Job drawing, mm, ordinate dimensions from the low corner. One solid piece. A direction names the side the tool comes from. Coordinates: 2 decimals unless noted, no trailing zeros. Order: outer loops, then holes, each group sorted by start corner. A loop starts at its lowest first (then second) coordinate and runs counter-clockwise, first axis right, second up. Notation, with made-up numbers: (26, -26) - (52, -26) arc R18 cw to (52, -2) - close; hole circle Ø6 at (37.25, 11). An arc over 180 degrees is marked (long way). Use one line per item in the form item = value.
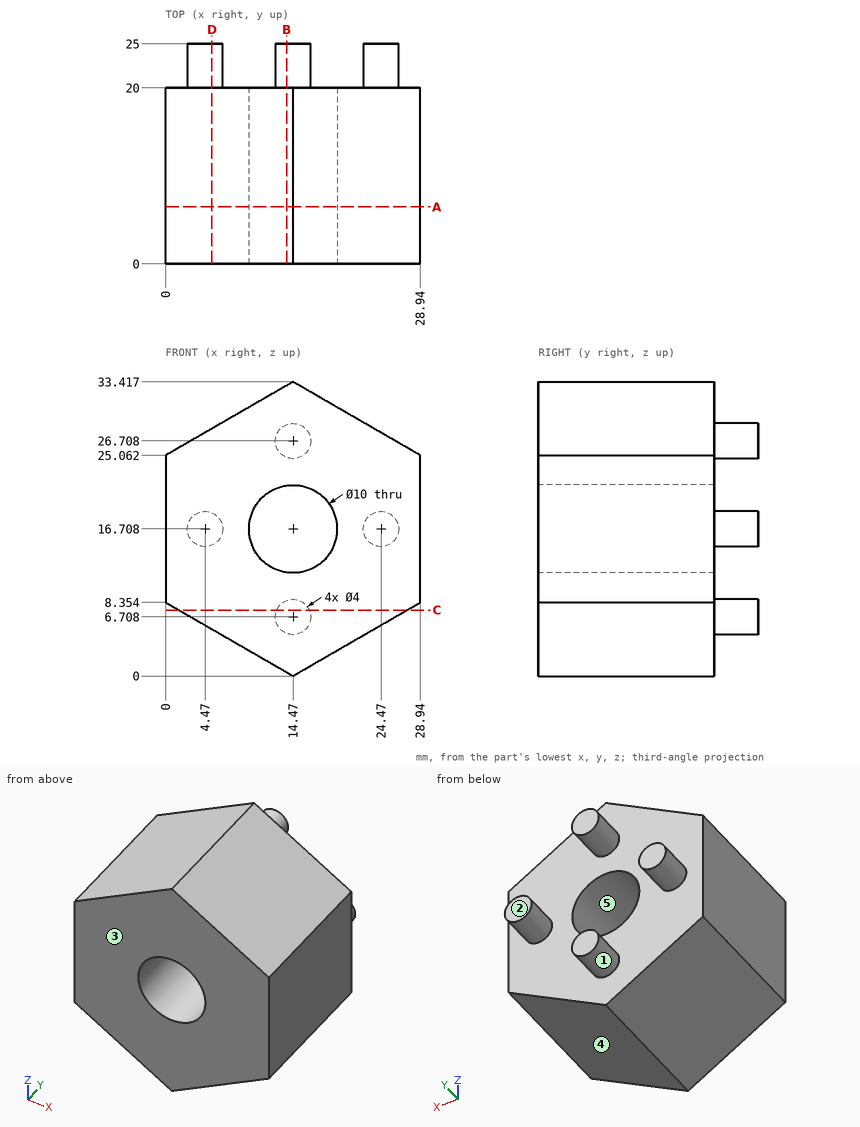
Item 1: Cut at B-B, the plane x = 13.75. Write the cut outline in (y, z) (1 decimal).
Derived:
outline = (0, 0.4) - (20, 0.4) - (20, 4.8) - (25, 4.8) - (25, 8.6) - (20, 8.6) - (20, 11.8) - (0, 11.8) - close; (0, 21.7) - (20, 21.7) - (20, 24.8) - (25, 24.8) - (25, 28.6) - (20, 28.6) - (20, 33) - (0, 33) - close
Item 2: Two-plate mould, pull along Z, no slides. Class the marked faces 3, 4 and 5: +Z half, -Z half, draft (parallel to the pull), parting line (faces both ways), or undercut.
Derived:
face_3 = draft
face_4 = -Z half
face_5 = undercut
Item 3: Drill centre lines: line 1 (Y direction, x = 14.5, z = 31.5); line 2 (Z direction, x = 15.5, y = 10.5) (1 decimal); line 3 (Z direction, x = 24.5, y = 9.5) (1 decimal). Where is each one in solid material? Low to high. Write a range as [from, to].
Derived:
line_1 = [0, 20]
line_2 = [0.6, 11.8], [21.6, 32.8]
line_3 = [5.8, 27.6]
Item 4: Cut at D-D, the plane x = 5.25. Write the cut outline in (y, z).
Derived:
outline = (0, 5.32) - (20, 5.32) - (20, 14.87) - (25, 14.87) - (25, 18.55) - (20, 18.55) - (20, 28.09) - (0, 28.09) - close
Item 5: Cut at A-A, the plane y = 6.5. Write the cut outline in (x, z) (1 decimal).
Derived:
outline = (0, 8.4) - (14.5, 0) - (28.9, 8.4) - (28.9, 25.1) - (14.5, 33.4) - (0, 25.1) - close; hole circle Ø10 at (14.5, 16.7)
Item 6: 3-axis set-ups, long thin cutter, end or side, ignore diameter. For the marked faces 1 and 2: which of +Z, -Z, +X, -X, +Y, -Y reach the whole face in a straight line?
Derived:
face_1 = +Y
face_2 = +Z, -Z, +X, -X, +Y
Item 7: Drop flat-ended pins along their axis: pin 1 (1 mm diameter, centred on x = 11.5, y = 10, fed in from +Z); pin 2 (5 mm diameter, centred on x = 21, y = 5, fed in from +Z); pin 3 (11.5 mm diameter, centred on x = 14.47, z = 16.71, fed in from -Y); pin 4 (1 mm diameter, centred on x = 17, z = 8, fed in from +Y). Give the stop position or say it passes through.
Derived:
pin_1 = 31.99
pin_2 = 31.09
pin_3 = 0
pin_4 = 20
Item 8: Cut at C-C, the plane z = 7.5. Write the cut outline in (x, y).
Derived:
outline = (1.48, 0) - (27.46, 0) - (27.46, 20) - (16.31, 20) - (16.31, 25) - (12.63, 25) - (12.63, 20) - (1.48, 20) - close
